from build123d import *

# Parameters (mm, degrees)
F0_W     = 20
F0_H     = 5
F1_DEPTH = 5
F3_DEPTH = 27.5
F4_DEPTH = 7.5
F5_W     = 4.5
F5_H     = 5
F6_DEPTH = 9.5
F7_W     = 4.5
F7_H     = 5
F8_DEPTH = 9.5


with BuildPart() as f1:
    # F0 (on Front) → F1 (new body)
    with BuildSketch(Plane.XZ):
        Polygon((-75.340211, 45), (-75.340211, 0), (64.659789, 0), (64.659789, 45), (44.659789, 45), (44.659789, 40), (24.659789, 40), (24.659789, 45), (-15.340211, 45), (-15.340211, 40), (-35.340211, 40), (-35.340211, 45), align=None)
        Polygon((14.659789, 5), (-55.340211, 5), (-65.340211, 5), (-65.340211, 10), (-55.340211, 10), (14.659789, 10), align=None, mode=Mode.SUBTRACT)
        with Locations((-25.340211, 32.5)):
            Rectangle(F0_W, F0_H, mode=Mode.SUBTRACT)
        with Locations((34.659789, 32.5)):
            Rectangle(F0_W, F0_H, mode=Mode.SUBTRACT)
    extrude(amount=F1_DEPTH)

    # F0 (on Front) → F3 (join)
    with BuildSketch(Plane.XZ):
        with Locations((-25.340211, 42.5)):
            Rectangle(F0_W, F0_H)
        with Locations((34.659789, 42.5)):
            Rectangle(F0_W, F0_H)
    extrude(amount=F3_DEPTH)

    # F2 (on face) → F4 (join)
    with BuildSketch(Plane.XZ.offset(5)):
        Polygon((-35.340211, 45), (-75.340211, 45), (-75.340211, 35), (-35.340211, 35), (-15.340211, 35), (24.659789, 35), (44.659789, 35), (64.659789, 35), (64.659789, 45), (44.659789, 45), (44.659789, 40), (24.659789, 40), (24.659789, 45), (-15.340211, 45), (-15.340211, 40), (-35.340211, 40), align=None)
    extrude(amount=F4_DEPTH)

    # F5 (on face) → F6 (join)
    with BuildSketch(Plane.XZ.offset(27.5)):
        with Locations((-37.590211, 42.5)):
            Rectangle(F5_W, F5_H)
        with Locations((-13.090211, 42.5)):
            Rectangle(F5_W, F5_H)
    extrude(amount=-F6_DEPTH)

    # F7 (on face) → F8 (join)
    with BuildSketch(Plane.XZ.offset(27.5)):
        with Locations((22.409789, 42.5)):
            Rectangle(F7_W, F7_H)
        with Locations((46.909789, 42.5)):
            Rectangle(F7_W, F7_H)
    extrude(amount=-F8_DEPTH)


solid = f1.part
Input: part model. Units: mm. Frame: model coordinates. A direction names the side the tool comes from. Give positions to 0.01 mm unless a question says otherwise; leave off trailing zeros. Write each loop counter-clockwise with the first axis right and the second up, starting at its lowest first coordinate (ties: lowest second). Pieces come first, ordered by that corner, then holes. Notation, with made-up numbers: (-13, -1.5) -> (-7, -1.5) arc R7 ccw to (-7, 5.5) -> close; hole circle Ø3 at (-31.75, 32). An arc over 180 degrees is marked (long way). Use one line per item in the form item = value. Start each with the question number.
1) Section query A-A on z = 7. Return the cut outline in (x, y).
2) Ray query, probe 1 along Z at (x, y) = (-3.5, -2.5); probe 2 along Y at (x, z) = (30, 16.5); probe 3 along Z at (x, y) = (42.5, -19). Return the intervals inside material, ascending. Write a range as from..to.
3) Section query C-C on y = -2. Return the cut outline in (x, z), then the cut area to 3 significant figures.
4) Section query D-D on x = -20. Return the cut outline in (y, z), then the cut area to 3 significant figures.
5) Set-up query: faces 5 (the flat face through (34, -20, 40)), 6 (the flat face through (-35.34, -15, 42)), 7 (the flat face through (-6, -8, 35)). Return all of +Z, -Z, +X, -X, +Y, -Y with unobstructed straight access to the full face (end or side cutting, diameter ignored); none if empty.
6) Draft query along X for faces 1 (the flat face through (-38, -18, 43)), 2 (the flat face through (44.66, -2, 32)), 3 (the flat face through (-25, -2, 5)), 4 (the flat face through (64.66, -3, 27)). Return one class per face: pulls with the +X half, pulls with the -X half, needs draft (parallel to the pull), parting line crosses it, or undercut.
7) Section query B-B on x = -6. Return the cut outline in (y, z), then the cut area to 3 significant figures.
8) Pin query (flat end, axial travel): pin 1 (1.5 mm diameter, centred on y = -22, z = 42.5, fed in from +X); pin 2 (1 mm diameter, centred on x = 29, z = 25, fed in from -Y); pin 3 (4 mm diameter, centred on y = -23, z = 42.5, fed in from -X). Return the tip coordinate at first contact, or that it passes through.
Outcome:
q1.outline = (-75.34, -5) -> (-65.34, -5) -> (-65.34, 0) -> (-75.34, 0) -> close; (14.66, -5) -> (64.66, -5) -> (64.66, 0) -> (14.66, 0) -> close
q2.probe_1 = 0..5, 10..45
q2.probe_2 = -5..0
q2.probe_3 = 40..45
q3.outline = (-75.34, 0) -> (64.66, 0) -> (64.66, 45) -> (-75.34, 45) -> close; hole (-65.34, 5) -> (14.66, 5) -> (14.66, 10) -> (-65.34, 10) -> close; hole (-35.34, 30) -> (-15.34, 30) -> (-15.34, 35) -> (-35.34, 35) -> close; hole (24.66, 30) -> (44.66, 30) -> (44.66, 35) -> (24.66, 35) -> close
q3.area = 5,700 mm^2
q4.outline = (-27.5, 40) -> (-12.5, 40) -> (-12.5, 35) -> (0, 35) -> (0, 45) -> (-27.5, 45) -> close; (-5, 0) -> (0, 0) -> (0, 5) -> (-5, 5) -> close; (-5, 10) -> (0, 10) -> (0, 30) -> (-5, 30) -> close
q4.area = 325 mm^2
q5.face_5 = -Z, +X, -X, -Y
q5.face_6 = +Z, -Z, -X
q5.face_7 = -Y
q6.face_1 = needs draft
q6.face_2 = undercut
q6.face_3 = undercut
q6.face_4 = pulls with the +X half
q7.outline = (-12.5, 35) -> (-5, 35) -> (-5, 10) -> (0, 10) -> (0, 45) -> (-12.5, 45) -> close; (-5, 0) -> (0, 0) -> (0, 5) -> (-5, 5) -> close
q7.area = 275 mm^2
q8.pin_1 = 49.16
q8.pin_2 = -5
q8.pin_3 = -39.84
